```python
from build123d import *

# Parameters (mm, degrees)
CORTE_EXTRUS_O1_DEPTH = 4
FILETE1_R             = 0.25
FILETE2_R             = 0.25


with BuildPart() as part:
    # Esboço1 → Revolução1 (revolve)
    with BuildSketch(Plane.XY):
        Polygon((-7.322649731, 3), (-7.122649731, 3), (-6.833974596, 3.5), (-6.433974596, 3.5), (-6.145299462, 3), (-2.5, 3), (-2.5, 4), (1.5, 4), (1.5, 2.25), (7.5, 2.25), (7.5, 1.75), (-3.200961894, 1.75), (-4.5, 2.5), (-8.5, 2.5), (-8.5, 3), (-8.3, 3), (-8.011324865, 3.5), (-7.611324865, 3.5), align=None)
    revolve(axis=Axis((-29.721905334, 0, 0), (1, 0, 0)))

    # Esboço2 → Corte-extrusão1 (cut)
    with BuildSketch(Plane(origin=(1.5, 0, 0), x_dir=(0, 0, -1), z_dir=(1, 0, 0))):
        with BuildLine():
            Line((-2, 3.464101615), (2, 3.464101615))
            ThreePointArc((2, 3.464101615), (0, 4), (-2, 3.464101615))
        make_face()
        with BuildLine():
            Line((-4, 0), (-2, 3.464101615))
            ThreePointArc((-2, 3.464101615), (-3.464101615, 2), (-4, 0))
        make_face()
        with BuildLine():
            ThreePointArc((-4, 0), (-3.464101615, -2), (-2, -3.464101615))
            Line((-2, -3.464101615), (-4, 0))
        make_face()
        with BuildLine():
            ThreePointArc((-2, -3.464101615), (0, -4), (2, -3.464101615))
            Line((2, -3.464101615), (-2, -3.464101615))
        make_face()
        with BuildLine():
            ThreePointArc((2, -3.464101615), (3.464101615, -2), (4, 0))
            Line((4, 0), (2, -3.464101615))
        make_face()
        with BuildLine():
            Line((2, 3.464101615), (4, 0))
            ThreePointArc((4, 0), (3.464101615, 2), (2, 3.464101615))
        make_face()
    extrude(amount=-CORTE_EXTRUS_O1_DEPTH, mode=Mode.SUBTRACT)

    # Filete1
    filete1_edges = [part.edges().sort_by_distance(p)[0] for p in [
        (-8.011324865, -3.5, 0),
        (-7.611324865, -3.5, 0),
    ]]
    fillet(filete1_edges, radius=FILETE1_R)

    # Filete2
    filete2_edges = [part.edges().sort_by_distance(p)[0] for p in [
        (-6.833974596, -3.5, 0),
        (-6.433974596, -3.5, 0),
    ]]
    fillet(filete2_edges, radius=FILETE2_R)


solid = part.part
```
Model file for the job. Use its own axes, mm. A direction names the side the tool comes from. Coordinates: 2 decimals unless noted, no trailing zeros. Loops run counter-clockwise (first coordinate to the right, second up) from the corner with the lowest first, then second, coordinate; pieces in that order, holes last. Notation, with made-up numbers: (3.5, 5.25) - (11.5, 5.25) arc R23 cw to (11.5, 36.25) - close; hole circle Ø4 at (12.25, -13). An arc over 180 degrees is marked (long way). Write item = value, one per line. Start each with the question number.
Item 1: 3-axis set-ups, long thin cutter, end or side, ignore diameter. For faces 5 (the face through (-0.472, 1.756, -2.986)), 6 (the face through (1.5, -2, -2)), 7 (the face through (-0.472, -1.756, 2.986)): which of +Z, -Z, +X, -X, +Y, -Y reach the whole face in a straight line?
Item 2: Wall check: probe 1 along Z at (x, y) = (-5.5, 0); probe 2 along X at (y, z) = (1, -2.5); probe 3 along Z at (x, y) = (-6.65, 0). Give the ranges that are in metal, low to high. Write a range as [from, to].
Item 3: Pull direction Z, two halves, no side cores. Call faces 1 (the face through (-0.472, 1.708, 3.014)), 2 (the face through (-0.472, -1.708, -3.014)), 3 (the face through (2.075, 1.617, -0.67)), 4 (the face through (-8.5, 2, 2)): +Z half, -Z half, draft (parallel to the pull), parting line (faces both ways), or undercut.
Item 4: Saw through at B-B, the plane x = -3. List the corners of the cut face in (y, z), then the cut area to 3 significant figures.
Item 5: Saw through at C-C, the plane x = 6. List the corners of the cut face in (y, z), then the cut area to 3 significant figures.
Item 6: Saw through at A-A, the plane x = 0.25. List the corners of the cut face in (y, z), then the cut area to 3 significant figures.
Item 7: Drop flat-ended pins along their axis: pin 1 Ø4 at (x, y) = (4.5, 2) entering from +Z; pin 2 Ø3 at (x, z) = (-1, 0.5) entering from -Y; pin 3 Ø1.2 at (x, z) = (-1, 0.5) entering from +Y. Give the stop position or say it passes through.
Answers:
q1.face_5 = -Z, +X, +Y
q1.face_6 = +X
q1.face_7 = +Z, +X, -Y
q2.probe_1 = [-3, -2.5], [2.5, 3]
q2.probe_2 = [-8.5, 1.5]
q2.probe_3 = [-3.5, -2.5], [2.5, 3.5]
q3.face_1 = +Z half
q3.face_2 = -Z half
q3.face_3 = undercut
q3.face_4 = draft
q4.outline = circle Ø6 at (0, 0); hole circle Ø3.5 at (0, 0)
q4.area = 18.7 mm2
q5.outline = circle Ø4.5 at (0, 0); hole circle Ø3.5 at (0, 0)
q5.area = 6.28 mm2
q6.outline = (-3.46, -2) - (0, -4) - (3.46, -2) - (3.46, 2) - (0, 4) - (-3.46, 2) - close; hole circle Ø3.5 at (0, 0)
q6.area = 31.9 mm2
q7.pin_1 = 2.25
q7.pin_2 = -3.46
q7.pin_3 = 3.46
